Part model, mm, in its own coordinate system. A direction names the side the tool comes from. Give positions to 0.01 mm unless a question says otherwise; leave off trailing zeros. Write each loop counter-clockwise with the first axis right and the second up, starting at its lowest first coordinate (ties: lowest second). Pieces come first, ordered by that corner, then holes.
Autodesk Inventor part; units mm, degrees
ref_plane "YZ Plane" through (0, 0, 0) normal (1, 0, 0) x (0, 1, 0)
ref_plane "XZ Plane" through (0, 0, 0) normal (0, 1, 0) x (-1, 0, 0)
ref_plane "XY Plane" through (0, 0, 0) normal (0, 0, 1) x (1, 0, 0)
sketch "Szkic1" plane through (0, 0, 0) normal (0, 1, 0) x (-1, 0, 0)
  line L0 (0, 0) -> (0, -49.4)
  line L1 (0, 0) -> (108, 0)
  line L2 (0, 0) -> (108.995, 0)
  line L3 (108.995, 0) -> (108.995, -49.4)
  line L4 (108.995, -49.4) -> (0, -49.4)
  line L5 (0, -49.4) -> (0, 0)
  line L6 (0, 0) -> (0, 2)
  line L7 (0, 2) -> (-2, 2)
  line L8 (108.995, -49.4) -> (110.995, -49.4)
  line L9 (110.995, -49.4) -> (110.995, -51.4)
  line L10 (110.995, -51.4) -> (-2, -51.4)
  line L11 (-2, -51.4) -> (-2, 2)
  line L12 (-2, 2) -> (110.995, 2)
  line L13 (110.995, 2) -> (110.995, -51.4)
  line L14 (110.995, 2) -> (100.995, 2)
  line L15 (100.995, 2) -> (100.995, 0)
  line L16 (110.995, -51.4) -> (100.995, -51.4)
  line L17 (100.995, -51.4) -> (100.995, -49.4)
  line L18 (-2, 2) -> (8, 2)
  line L19 (8, 2) -> (8, 0)
  line L20 (-2, -51.4) -> (8, -51.4)
  line L21 (8, -51.4) -> (8, -49.4)
  line L22 (-2, 0) -> (0, 0)
  line L23 (108.995, 0) -> (110.995, 0)
  line L24 (108.995, -49.4) -> (110.995, -49.4)
  line L25 (-2, -49.4) -> (0, -49.4)
  line L26 (100.995, 2) -> (90.995, 2)
  line L27 (90.995, 2) -> (90.995, 0)
  line L28 (100.995, -51.4) -> (90.995, -51.4)
  line L29 (90.995, -51.4) -> (90.995, -49.4)
  line L30 (110.995, -24.7) -> (-2, -24.7)
  line L31 (54.4975, -51.4) -> (54.4975, 2)
  line L32 (90.995, 2) -> (60.995, 2)
  line L33 (60.995, 2) -> (60.995, 0)
  line L34 (48, 2) -> (48, 0)
  line L35 (60.995, -51.4) -> (60.995, -49.4)
  line L36 (48, -51.4) -> (48, -49.4)
  point P0 (48, 0)
  dimension "d0" = 49.4
  dimension "d1" = 108
  dimension "d2" = 2
  dimension "d3" = 2
  dimension "d4" = 2
  dimension "d5" = 2
  dimension "d6" = 10
  dimension "d7" = 10
  dimension "d8" = 10
  dimension "d9" = 10
  dimension "d16" = 10
  dimension "d17" = 10
  dimension "d33" = 30
extrude "Wyciągnięcie proste1" add sketch "Szkic1" along normal blind 20 contours L6 L12 L19 L1 | L22 L11 L7 L6 | L19 L12 L34 L1 | L4 L21 L10 L11 L25 | L34 L12 L31 L1 | L4 L36 L10 L21 | L31 L10 L36 L4 | L4 L35 L10 L31 | L31 L12 L33 L1 | L2 L1 L15 L12 L13 L23 | L8 L9 L10 L17 L4 | L4 L29 L10 L35 | L33 L12 L27 L1 | L17 L10 L29 L4 | L27 L12 L15 L1
sketch "Szkic2" plane through (0, 20, 0) normal (0, 1, 0) x (1, 0, 0)
  line L0 (-8, -2) -> (2, -2)
  line L1 (2, 51.4) -> (-110.995, 51.4)
  line L2 (2, -2) -> (-110.995, -2)
  line L3 (-110.995, -2) -> (-110.995, 51.4)
  line L4 (-110.995, 51.4) -> (2, 51.4)
  line L5 (2, 51.4) -> (2, -2)
  line L6 (-110.995, 0) -> (-110.995, 10)
  line L7 (-110.995, 49.4) -> (2, 49.4)
  line L8 (-110.995, 49.4) -> (-110.995, 39.4)
  arc A0 (-110.995, 10) -> (-110.995, 39.4) centre (-125.3914, 24.7) ccw
  arc A1 (-110.995, 10) -> (-110.995, 39.4) centre (-108.7482, 24.7) ccw
  point P0 (0, 0)
  point P1 (-100.995, 51.4)
  point P2 (-100.995, 49.4)
  point P3 (-100.995, 51.4)
  point P4 (-90.995, 51.4)
  point P5 (-90.995, 49.4)
  point P6 (-60.995, 51.4)
  point P7 (-60.995, 49.4)
  dimension "d12" = 10
  dimension "d13" = 10
extrude "Wyciągnięcie proste2" add sketch "Szkic2" along normal blind 5 contours L2 L3 A1 L7 L5 L0 | L7 L3 L1 L5
sketch "Szkic3" plane through (2, 0, -49.4) normal (1, 0, 0) x (0, 0, -1)
  line L0 (-39.4, 25) -> (-51.4, 25)
  line L1 (2, 0) -> (2, 20)
  line L2 (-51.4, 25) -> (2, 25)
  line L3 (2, 25) -> (2, 15)
  line L4 (2, 15) -> (-51.4, 15)
  line L5 (-51.4, 15) -> (-51.4, 25)
  point P0 (-49.4, 0)
  dimension "d18" = 10
extrude "Wyciągnięcie proste3" add sketch "Szkic3" against normal blind 1
chamfer "Faza1" distance 6 angle 45 2 edges at (1.5, 15, 0) (1.5, 15, -49.4)
sketch "Szkic5" plane through (0, 25, 0) normal (0, 1, 0) x (1, 0, 0)
  line L0 (-110.995, -2) -> (2, -2)
  line L1 (2, -2) -> (2, 7)
  line L2 (2, -2) -> (11, -2) construction
  line L3 (2, 7) -> (-12.5, 7)
  line L4 (-54.4975, -2) -> (-54.4975, 51.4)
  line L5 (2, 51.4) -> (-110.995, 51.4)
  line L6 (2, -2) -> (2, 51.4)
  line L7 (2, 24.7) -> (-94.0806, 24.7)
  line L8 (-110.995, 7) -> (-96.495, 7)
  line L9 (2, 42.4) -> (-12.5, 42.4)
  line L10 (-110.995, 42.4) -> (-96.495, 42.4)
  line L11 (-12.5, 7) -> (-82.5, 7) construction
  line L12 (-12.5, 9.5) -> (-82.5, 9.5)
  line L13 (-82.5, 4.5) -> (-12.5, 4.5)
  arc A0 (-12.5, 4.5) -> (-12.5, 9.5) centre (-12.5, 7) ccw
  arc A1 (-82.5, 9.5) -> (-82.5, 4.5) centre (-82.5, 7) ccw
  line L14 (-12.5, 42.4) -> (-82.5, 42.4) construction
  line L15 (-12.5, 44.9) -> (-82.5, 44.9)
  line L16 (-82.5, 39.9) -> (-12.5, 39.9)
  arc A2 (-12.5, 39.9) -> (-12.5, 44.9) centre (-12.5, 42.4) ccw
  arc A3 (-82.5, 44.9) -> (-82.5, 39.9) centre (-82.5, 42.4) ccw
  line L17 (-12.5, 42.4) -> (57.5, 42.4) construction
  point P0 (0, 0)
  point P1 (-47.5, 7)
  point P2 (-47.5, 42.4)
  dimension "d37" = 9
  dimension "d38" = 90
  dimension "d39" = 14.5
  dimension "d40" = 70
  dimension "d41" = 5
  dimension "d42" = 70
  dimension "d43" = 180
  dimension "d44" = 5
extrude "Wyciągnięcie proste5" cut sketch "Szkic5" against normal blind 20 contours L13 A1 L12 L4 | L4 L12 A0 L13 | L16 A3 L15 L4 | L4 L15 A2 L16
properties part number "klapa"
1) Wall check: L1, parallel to Z at x = -60.5, y = 6.25; L2, parallel to Y at x = -5, z = -30; L3, parallel to X at y = 15.5, z = -33.5. Give the ranges that are in metal, low to high.
Answers follow:
L1: z = -51.4 to -49.4, 0 to 2
L2: y = 20 to 25
L3: x = 1 to 2
2) Saw through at D-D, the plane z = -24.7. Write the cut outline in (x, y).
Answers follow:
outline: (-93.88, 20) - (1, 20) - (1, 15) - (2, 15) - (2, 25) - (-93.88, 25) - close
3) Pin check, flat tips, straight feed: pin 1 Ø8 at (x, z) = (-74, -33.5) entering from -Y; pin 2 Ø3.5 at (y, z) = (15, -36.5) entering from -X; pin 3 Ø0.8 at (x, z) = (1.5, -20.5) entering from -Y. Stop position of each tip, or through.
Answers follow:
pin 1: stops at y = 20
pin 2: stops at x = 1
pin 3: stops at y = 15
4) Two-plate mould, pull along X, no slides. Class faces 1 (the face through (-110.995, 18, -50)), 2 (the face through (-10, 22.5, -42.3)), 3 (the face through (-47, 23, -9.5)), 4 (the face through (-54, 12, 2)): +X half, -X half, draft (parallel to the pull), parting line (faces both ways), or undercut.
Answers follow:
face 1: -X half
face 2: undercut
face 3: undercut
face 4: draft
5) 3-axis set-ups, long thin cutter, end or side, ignore diameter. For faces 5 (the face through (1.5, 12, -3)), 6 (the face through (-55, 10, -49.4)), 7 (the face through (-54, 12, -51.4)), 8 (the face through (-110.995, 18, 1)), 9 (the face through (-85, 22.5, -42.5)): which of +Z, -Z, +X, -X, +Y, -Y reach the whole face in a straight line?
Answers follow:
face 5: +X, -X, -Y
face 6: -X, -Y
face 7: -Z, +X, -X, +Y, -Y
face 8: +Z, -Z, -X, +Y, -Y
face 9: +Y, -Y
6) Saw through at A-A, the plane y = 10.75. Write the cut outline in (x, z) (3 decimals), then the cut area to 3 significant figures.
Answers follow:
outline: (-110.995, -51.4) - (2, -51.4) - (2, -47.65) - (1, -47.65) - (1, -49.4) - (-110.995, -49.4) - close; (-110.995, 0) - (1, 0) - (1, -1.75) - (2, -1.75) - (2, 2) - (-110.995, 2) - close
area: 455 mm2
7) Saw through at C-C, the plane x = -97. Write the cut outline in (y, z).
Answers follow:
outline: (0, -51.4) - (25, -51.4) - (25, -33.82) - (20, -33.82) - (20, -49.4) - (0, -49.4) - close; (0, 0) - (20, 0) - (20, -15.58) - (25, -15.58) - (25, 2) - (0, 2) - close
8) Saw through at B-B, the plane x = -57.5. Write the cut outline in (y, z).
Answers follow:
outline: (0, -51.4) - (25, -51.4) - (25, -44.9) - (20, -44.9) - (20, -49.4) - (0, -49.4) - close; (0, 0) - (20, 0) - (20, -4.5) - (25, -4.5) - (25, 2) - (0, 2) - close; (20, -39.9) - (25, -39.9) - (25, -9.5) - (20, -9.5) - close
